For this review, use the dimensioned drawing (mm, ordinates from the lowest corner) and the shaded views. A direction names the side the tool comes from. Round coordinates to 2 decimals unless told otherwise and drop trailing zeros. Write each loop counter-clockwise with the first axis right and the second up, starting at its lowest first coordinate (ties: lowest second). Pieces come first, ordered by that corner, then holes.
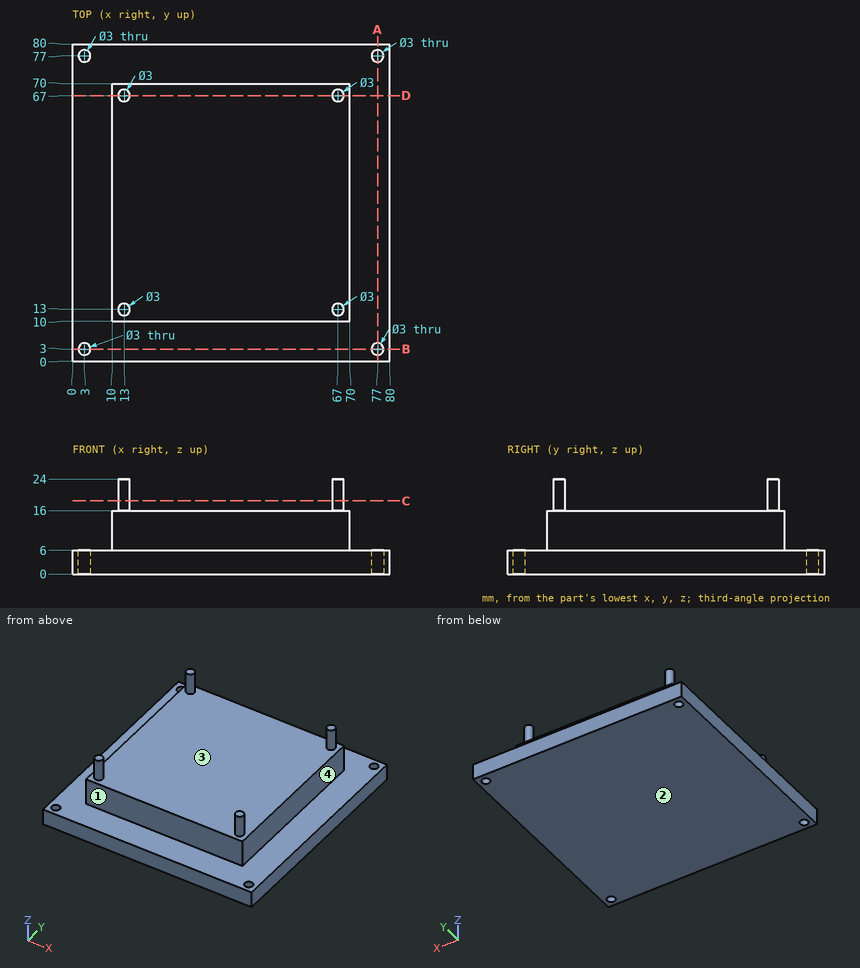
1) Add section A-A on x = 77. State the section outline as (y, z) points, and give its area (3 significant figures).
2) Add section C-C on z = 18.5. State the section outline as (x, y) points.
3) Add section D-D on y = 67. State the section outline as (x, z) points, and give its area (3 significant figures).
4) For line 1 along X through (y, z) = (77, 3.35); line 2 along Y through (x, z) = (65.5, 11.25), list the stretches that pass through material, from the lowest coordinate up.
5) For P1, Ø2.5, axis at x = 3, y = 77, coming from the +Z side; P2, Ø6, axis at x = 68.5, z = 13.5, coming from the -Y side; P3, Ø5, axis at x = 38, y = 29, coming from the +Z side; P4, Ø5, axis at y = 51.5, z = 9.5, coming from the -X side, all flat-tipped, find the tip position at first contact; note any pin that passes through.
6) For the marked faces 1, 2, 3 and 4, list the 3-axis set-ups (+Z, -Z, +X, -X, +Y, -Y) from which the entire face can be reached by the end or side of a thin tool; tool diameter is ignored.
Computed:
1. outline: (0, 0) - (1.5, 0) - (1.5, 6) - (0, 6) - close; (4.5, 0) - (75.5, 0) - (75.5, 6) - (4.5, 6) - close; (78.5, 0) - (80, 0) - (80, 6) - (78.5, 6) - close
1. area: 444 mm2
2. outline: circle Ø3 at (13, 13); circle Ø3 at (13, 67); circle Ø3 at (67, 13); circle Ø3 at (67, 67)
3. outline: (0, 0) - (80, 0) - (80, 6) - (70, 6) - (70, 16) - (68.5, 16) - (68.5, 24) - (65.5, 24) - (65.5, 16) - (14.5, 16) - (14.5, 24) - (11.5, 24) - (11.5, 16) - (10, 16) - (10, 6) - (0, 6) - close
3. area: 1,130 mm2
4. line 1: x = 0 to 1.5, 4.5 to 75.5, 78.5 to 80
4. line 2: y = 10 to 70
5. P1: passes through
5. P2: stops at y = 10
5. P3: stops at z = 16
5. P4: stops at x = 10
6. face 1: +Z, +X, -X, -Y
6. face 2: -Z, +X, -X, +Y, -Y
6. face 3: +Z
6. face 4: +Z, +X, +Y, -Y
